```python
from build123d import *

# Parameters (mm, degrees)
SKETCH1_R           = 4.7625
BOSS_EXTRUDE1_DEPTH = 3.175
SKETCH2_R           = 3.96875
BOSS_EXTRUDE2_DEPTH = 4.7625
SKETCH3_R           = 1.5875
CUT_EXTRUDE1_DEPTH  = 11.409933657


with BuildPart() as part:
    # Sketch1 → Boss-Extrude1 (new body)
    with BuildSketch(Plane.XY):
        Circle(SKETCH1_R)
    extrude(amount=BOSS_EXTRUDE1_DEPTH)

    # Sketch2 → Boss-Extrude2 (add)
    with BuildSketch(Plane.XY.offset(3.175)):
        with Locations(Location((0, 0, 0), (0, 0, 180))):
            Circle(SKETCH2_R)
    extrude(amount=BOSS_EXTRUDE2_DEPTH)

    # Sketch3 → Cut-Extrude1 (cut, through all)
    with BuildSketch(Plane.XY.offset(7.9375)):
        Circle(SKETCH3_R)
    extrude(amount=-CUT_EXTRUDE1_DEPTH, mode=Mode.SUBTRACT)


solid = part.part
```
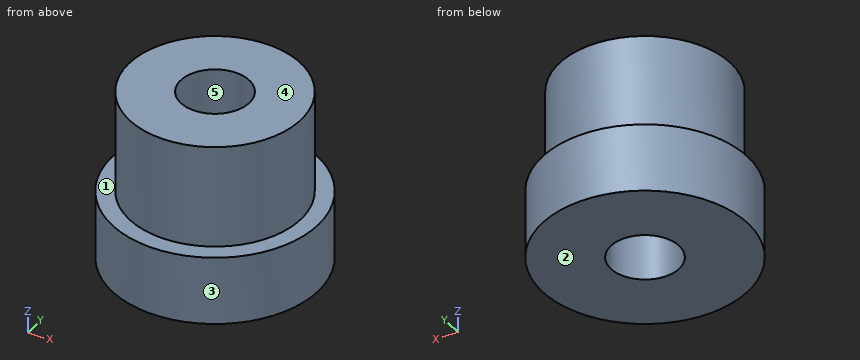
Verification items for the finished model (mm, model axes). Face numbers are marked on the shaded views. A direction names the side the tool comes from. Round coordinates to 2 decimals unless told otherwise and drop trailing zeros. Order: outer loops, then holes, each group sorted by start corner. A loop starts at its lowest first (then second) coordinate and runs counter-clockwise, first axis right, second up. Notation, with made-up numbers: (10.5, 69.5) -> (17.5, 69.5) arc R24 ccw to (17.5, 88.5) -> close; hole circle Ø2 at (63.25, -24.75). An arc over 180 degrees is marked (long way). Put each result on its own line as item: value. Start each with the question number.
(1) Tool access check on the marked faces 1 and 2. Record the directions out of +Z, -Z, +X, -X, +Y, -Y that give a thin tool (end or side, any length) a straight path to the whole face; none if there is none.
(2) Material ranges on line 1 along Y through (x, z) = (0, 2.5); line 2 along Y through (x, z) = (0, 4); line 3 along Z through (x, y) = (3.25, 2.5) (3 decimals), recorded low to high.
(3) Draft check along Y on the marked faces 3, 4 and 5. Enter one of: +Y half, -Y half, draft (parallel to the pull), parting line (faces both ways), or undercut.
(4) Section check C-C (x = -2). Enter the section's corners in (y, z) (1 decimal), then the cut area to 3 significant figures.
(5) Depth check by flat-ended pin: pin 1 Ø2 at (x, z) = (0.5, 6) entering from +Y; pin 2 Ø3 at (x, y) = (-0.5, -2) entering from -Z; pin 3 Ø4 at (x, z) = (3.5, 5.5) entering from -Y. Enter the tip coordinate at first touch or a pass-through.
(6) Section check D-D (z = 1.5). Enter the section's corners in (x, y) (1 decimal), then the cut area to 3 significant figures.
(7) Section check A-A (y = 0). Enter the section's corners in (x, z) (1 decimal).
Completed:
1. face 1: +Z
1. face 2: -Z, +X, -X, +Y, -Y
2. line 1: y = -4.76 to -1.59, 1.59 to 4.76
2. line 2: y = -3.97 to -1.59, 1.59 to 3.97
2. line 3: z = 0 to 3.175
3. face 3: parting line
3. face 4: draft
3. face 5: undercut
4. outline: (-4.3, 0) -> (4.3, 0) -> (4.3, 3.2) -> (3.4, 3.2) -> (3.4, 7.9) -> (-3.4, 7.9) -> (-3.4, 3.2) -> (-4.3, 3.2) -> close
4. area: 60.1 mm2
5. pin 1: stops at y = 3.97
5. pin 2: stops at z = 0
5. pin 3: stops at y = -3.67
6. outline: circle Ø9.5 at (0, 0); hole circle Ø3.2 at (0, 0)
6. area: 63.3 mm2
7. outline: (-4.8, 0) -> (-1.6, 0) -> (-1.6, 7.9) -> (-4, 7.9) -> (-4, 3.2) -> (-4.8, 3.2) -> close; (1.6, 0) -> (4.8, 0) -> (4.8, 3.2) -> (4, 3.2) -> (4, 7.9) -> (1.6, 7.9) -> close
